Part print with two shaded views. Sizes in mm from the minimum x, y, z corner. A direction names the side the tool comes from. Round coordinates to 2 decimals unless told otherwise and drop trailing zeros. Loops run counter-clockwise (first coordinate to the right, second up) from the corner with the lowest first, then second, coordinate; pieces in that order, holes last. Notation, with made-up numbers: M 48.25,25 L 90.25,25 A28 cw 90.25,54 Z; hole C 28,-24.75 d9. An arc over 180 degrees is marked long. Answer as CSV lines item,"result". Start each with the question number.
Item 1: Band-saw the part on C-C (y = 8.5). Give the cut face in (x, z), and give its area (3 significant figures).
Item 2: Band-saw the part on B-B (z = 60). Give the cut face in (x, y).
Item 3: Which spindle directions (+Z, -Z, +X, -X, +Y, -Y) get a long thin tool onto all of the face, cutting with end or side? Do the marked faces 4, 5 and 6. Say none if no direction does.
Item 4: Drop flat-ended pins along their axis: pin 1 Ø4 at (x, z) = (48, 16) entering from -Y; pin 2 Ø4 at (x, y) = (54.5, 17) entering from +Z; pin 3 Ø4 at (y, z) = (16, 18) entering from +X; pin 4 Ø7 at (x, z) = (60, 102) entering from +Y. Give the stop position or say it passes through.
Item 5: Band-saw the part on D-D (z = 18). Give the cut face in (x, y).
Item 6: Band-saw the part on A-A (x = 60). Give the cut face in (y, z), and give its area (3 significant figures).
Item 7: Mould opens along X. For the marked faces 1, 2 and 3 say: pulls with the +X half, pulls with the -X half, needs draft (parallel to the pull), parting line crosses it, or undercut.
Item 8: Wall check: line 1 (X direction, y = 10, z = 60); line 2 (X direction, y = 27.5, z = 60); line 3 (Y direction, x = 105.5, z = 72). Give the ranges that are in metal, low to high.
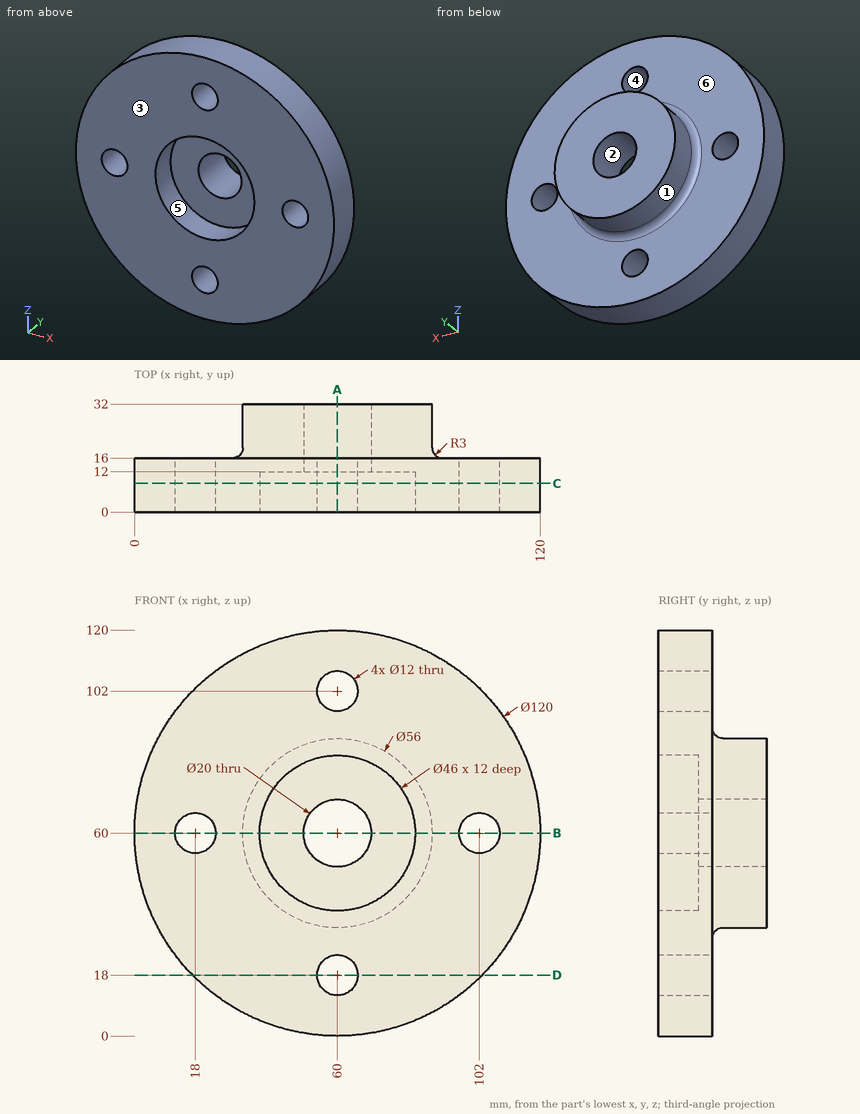
Answer block:
1,outline,"C 60,60 d120; hole C 18,60 d12; hole C 60,60 d46; hole C 60,18 d12; hole C 60,102 d12; hole C 102,60 d12"
1,area,"9,200 mm^2"
2,outline,"M 0,0 L 12,0 L 12,16 L 0,16 Z; M 24,0 L 37,0 L 37,12 L 50,12 L 50,32 L 32,32 L 32,19 A3 cw 29,16 L 24,16 Z; M 70,12 L 83,12 L 83,0 L 96,0 L 96,16 L 91,16 A3 cw 88,19 L 88,32 L 70,32 Z; M 108,0 L 120,0 L 120,16 L 108,16 Z"
3,face 4,"+Y, -Y"
3,face 5,"-Y"
3,face 6,"+Y"
4,pin 1,"stops at y = 0"
4,pin 2,"stops at z = 119.88"
4,pin 3,"stops at x = 104.72"
4,pin 4,"passes through"
5,outline,"M 17.15,0 L 54,0 L 54,16 L 17.15,16 Z; M 66,0 L 102.85,0 L 102.85,16 L 66,16 Z"
6,outline,"M 0,0 L 16,0 L 16,12 L 0,12 Z; M 0,24 L 16,24 L 16,29 A3 cw 19,32 L 32,32 L 32,50 L 12,50 L 12,37 L 0,37 Z; M 0,83 L 12,83 L 12,70 L 32,70 L 32,88 L 19,88 A3 cw 16,91 L 16,96 L 0,96 Z; M 0,108 L 16,108 L 16,120 L 0,120 Z"
6,area,"1,480 mm^2"
7,face 1,"parting line crosses it"
7,face 2,"undercut"
7,face 3,"needs draft"
8,line 1,"x = 0 to 12, 24 to 37, 83 to 96, 108 to 120"
8,line 2,"x = 32 to 50, 70 to 88"
8,line 3,"y = 0 to 16"
